```python
from build123d import *

# Parameters (mm, degrees)
CUT_EXTRUDE3_DEPTH           = 60
CUT_EXTRUDE5_DEPTH           = 2
CUT_EXTRUDE5_DEPTH_BACK      = 30
SKETCH9_R                    = 38
SKETCH9_R_2                  = 23
SKETCH19_W                   = 12
SKETCH19_H                   = 36.5
CUT_REVOLVE2_ANGLE           = 65
CUT_REVOLVE2_OTHER_WAY_ANGLE = 65
SKETCH21_W                   = 3.25
SKETCH21_H                   = 4
BOSS_EXTRUDE3_DEPTH          = 1.35
CIRPATTERN1_COUNT            = 5
CUT_EXTRUDE9_START           = -5
CUT_EXTRUDE9_DEPTH           = 5
SKETCH23_R                   = 10.5
CUT_EXTRUDE10_DEPTH          = 10
SKETCH24_W                   = 17
SKETCH24_H                   = 12
BOSS_EXTRUDE4_DEPTH          = 8
SKETCH26_W                   = 12
SKETCH26_H                   = 8
CUT_EXTRUDE11_DEPTH          = 10
SKETCH27_W                   = 4
SKETCH27_H                   = 5
CUT_EXTRUDE12_DEPTH          = 5
CUT_EXTRUDE14_DEPTH          = 2
CUT_EXTRUDE14_DEPTH_BACK     = 30
SKETCH29_R                   = 1
CUT_EXTRUDE15_DEPTH          = 15
FILLET1_R                    = 6
FILLET2_R                    = 8


# Read off the part's stored shape, not the designer's step: Cut-Extrude9
with BuildPart() as part:
    # Sketch1 → Revolve1 (revolve)
    with BuildSketch(Plane.XY, mode=Mode.PRIVATE) as revolve1_sk:
        with BuildLine():
            Line((0, 63.427876097), (32, 63.427876097))
            ThreePointArc((32, 63.427876097), (37.656854249, 61.084730346), (40, 55.427876097))
            Line((40, 55.427876097), (40, 28.846818009))
            ThreePointArc((40, 28.846818009), (38.792081772, 24.082439968), (35.460140376, 20.469057744))
            Line((35.460140376, 20.469057744), (28.539859624, 15.958818353))
            ThreePointArc((28.539859624, 15.958818353), (25.207918228, 12.345436129), (24, 7.581058088))
            Line((24, 7.581058088), (24, 3.25))
            Line((24, 3.25), (24.35, 3))
            Line((24.35, 3), (24.35, 0))
            Line((24.35, 0), (22.5, 0))
            Line((22.5, 0), (22.5, 12.5))
            ThreePointArc((22.5, 12.5), (22.353553391, 12.853553391), (22, 13))
            Line((22, 13), (0, 13))
            Line((0, 13), (0, 63.427876097))
        make_face()
    revolve(revolve1_sk.sketch.rotate(Axis((0, 0, 0), (0, 1, 0)), 90), axis=Axis((0, 0, 0), (0, 1, 0)))

    # Sketch11 → Cut-Extrude3 (cut)
    with BuildSketch(Plane(origin=(0, 13, 0), x_dir=(-1, 0, 0), z_dir=(0, -1, 0))):
        with BuildLine():
            Line((-21, 0), (21, 0))
            ThreePointArc((21, 0), (0, 21), (-21, 0))
        make_face()
    extrude(amount=-CUT_EXTRUDE3_DEPTH, mode=Mode.SUBTRACT)

    # Sketch9 → Cut-Extrude5 (cut, two sides: drawn at the far end of the back side and taken through both)
    with BuildSketch(Plane(origin=(0, 55.427876097, 0), x_dir=(1, 0, 0), z_dir=(0, 1, 0)).offset(-CUT_EXTRUDE5_DEPTH_BACK)):
        with Locations(Location((0, 0, 0), (0, 0, 270))):
            Circle(SKETCH9_R)
        with Locations(Location((0, 0, 0), (0, 0, 270))):
            Circle(SKETCH9_R_2, mode=Mode.SUBTRACT)
    extrude(amount=CUT_EXTRUDE5_DEPTH + CUT_EXTRUDE5_DEPTH_BACK, mode=Mode.SUBTRACT)

    # Sketch19 → Cut-Revolve2 (revolve, cut)
    with BuildSketch(Plane(origin=(0, 0, 0), x_dir=(0, 0, -1), z_dir=(1, 0, 0))):
        with Locations((-41.064715832, 37.177876097)):
            Rectangle(SKETCH19_W, SKETCH19_H)
    revolve(axis=Axis((0, 0, 0), (0, 1, 0)), revolution_arc=CUT_REVOLVE2_ANGLE, mode=Mode.SUBTRACT)

    # Sketch19 → Cut-Revolve2 other way (revolve, cut)
    with BuildSketch(Plane(origin=(0, 0, 0), x_dir=(0, 0, -1), z_dir=(1, 0, 0))):
        with Locations((-41.064715832, 37.177876097)):
            Rectangle(SKETCH19_W, SKETCH19_H)
    revolve(axis=Axis((0, 0, 0), (0, -1, 0)), revolution_arc=CUT_REVOLVE2_OTHER_WAY_ANGLE, mode=Mode.SUBTRACT)

    # Sketch21 → Boss-Extrude3 (add)
    with BuildSketch(Plane(origin=(0, 0, 22.5), x_dir=(-1, 0, 0), z_dir=(0, 0, -1))):
        with Locations((0, 2)):
            Rectangle(SKETCH21_W, SKETCH21_H)
    boss_extrude3 = extrude(amount=BOSS_EXTRUDE3_DEPTH)

    # CirPattern1: Boss-Extrude3 ×5 about axis
    cirpattern1_axis = Axis((0, 0, 0), (0, 1, 0))
    for i in range(1, CIRPATTERN1_COUNT):
        add(boss_extrude3.rotate(cirpattern1_axis, i * 360 / CIRPATTERN1_COUNT))

    # Cut-Extrude9 outline → Cut-Extrude9 (cut)
    with BuildSketch(Plane(origin=(0, 63.427876097, 0), x_dir=(1, 0, 0), z_dir=(0, 1, 0)).offset(CUT_EXTRUDE9_START)):
        with BuildLine():
            ThreePointArc((40, 0), (0, 40), (-40, 0))
            Line((-40, 0), (-21, 0))
            ThreePointArc((-21, 0), (0, 21), (21, 0))
            Line((21, 0), (40, 0))
        make_face()
    extrude(amount=CUT_EXTRUDE9_DEPTH, mode=Mode.SUBTRACT)

    # Sketch23 → Cut-Extrude10 (cut)
    with BuildSketch(Plane(origin=(0, 0, -40), x_dir=(-1, 0, 0), z_dir=(0, 0, -1))):
        with Locations((0, 42.137876097)):
            Circle(SKETCH23_R)
    extrude(amount=-CUT_EXTRUDE10_DEPTH, mode=Mode.SUBTRACT)

    # Sketch24 → Boss-Extrude4 (add)
    with BuildSketch(Plane(origin=(0, 58.427876097, 0), x_dir=(1, 0, 0), z_dir=(0, 1, 0))):
        with Locations((0, 30)):
            Rectangle(SKETCH24_W, SKETCH24_H)
    extrude(amount=-BOSS_EXTRUDE4_DEPTH)

    # Sketch26 → Cut-Extrude11 (cut)
    with BuildSketch(Plane(origin=(0, 58.427876097, 0), x_dir=(1, 0, 0), z_dir=(0, 1, 0))):
        with Locations((0, 30)):
            Rectangle(SKETCH26_W, SKETCH26_H)
    extrude(amount=-CUT_EXTRUDE11_DEPTH, mode=Mode.SUBTRACT)

    # Sketch27 → Cut-Extrude12 (cut)
    with BuildSketch(Plane(origin=(8.5, 0, 0), x_dir=(0, 0, -1), z_dir=(1, 0, 0))):
        with Locations((31, 53.927876097)):
            Rectangle(SKETCH27_W, SKETCH27_H)
    extrude(amount=-CUT_EXTRUDE12_DEPTH, mode=Mode.SUBTRACT)

    # Sketch28 → Cut-Extrude14 (cut, two sides: drawn at the far end of the back side and taken through both)
    with BuildSketch(Plane(origin=(0, 55.427876097, 0), x_dir=(1, 0, 0), z_dir=(0, 1, 0)).offset(-CUT_EXTRUDE14_DEPTH_BACK)):
        with BuildLine():
            Line((-22.912878475, -2), (22.912878475, -2))
            ThreePointArc((22.912878475, -2), (0, -23), (-22.912878475, -2))
        make_face()
    extrude(amount=CUT_EXTRUDE14_DEPTH + CUT_EXTRUDE14_DEPTH_BACK, mode=Mode.SUBTRACT)

    # Sketch29 → Cut-Extrude15 (cut)
    with BuildSketch(Plane(origin=(0, 0, 0), x_dir=(-1, 0, 0), z_dir=(0, 0, -1))):
        with Locations((-30.416198487, 60.927876097)):
            Circle(SKETCH29_R)
        with Locations((30.416198487, 60.927876097)):
            Circle(SKETCH29_R)
        with Locations((0, 60.927876097)):
            Circle(SKETCH29_R)
    extrude(amount=-CUT_EXTRUDE15_DEPTH, mode=Mode.SUBTRACT)

    # Fillet1
    fillet1_edges = [part.edges().sort_by_distance(p)[0] for p in [
        (21, 35.713938048, 0),
        (-21, 35.713938048, 0),
    ]]
    fillet(fillet1_edges, radius=FILLET1_R)

    # Fillet2
    fillet2_edges = [part.edges().sort_by_distance(p)[0] for p in [
        (-22.912878475, 41.427876097, 2),
        (22.912878475, 41.427876097, 2),
    ]]
    fillet(fillet2_edges, radius=FILLET2_R)


solid = part.part
```
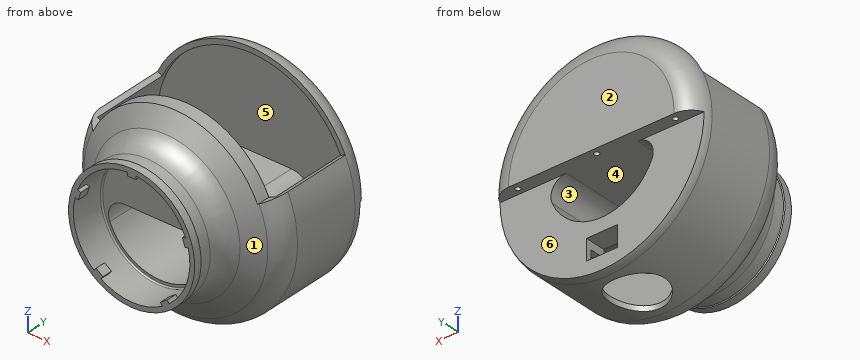
The listing builds one solid part. Answer for the finished solid, in the listing's coordinates (mm). Face numbers are marked on the shaded views. A direction names the side the tool comes from. Coordinates: 2 decimals unless noted, no trailing zeros. Write each loop counter-clockwise with the first axis right and the second up, starting at its lowest first coordinate (ties: lowest second). Pieces come first, ordered by that corner, then holes. Notation, with made-up numbers: (57, -34) - (101, -34) arc R30 ccw to (101, -9) - close; hole circle Ø6 at (57.5, 69). An arc over 180 degrees is marked (long way). Return JSON: item names as keys, results as strings. Group by question number.
Q1. The part is cut by section A-A on y = 22.5. Write down the section's boundary in (x, z), and give its area (3 significant figures).
Q2. The part is cut by section B-B on z = -1.5. State how many separate pieces and enclosed holes the cut face has, and give its area (3 significant figures).
Q3. Find the intervals of material crossed by line 1 along Y through (x, z) = (0, 8); line 2 along Y through (x, z) = (-9.5, 16); line 3 along X through (y, z) = (50, -9), in increasing order. Write a range as [from, to].
Q4. Flat-ended cylindrical pins translate along their axes: pin 1 Ø2 at (x, y) = (0, 61) entering from -Z; pin 2 Ø12 at (x, y) = (-19.5, 28) entering from -Z; pin 3 Ø10 at (x, z) = (2, 2.5) entering from -Y; pin 4 Ø13 at (x, z) = (-2, -27.5) entering from -Y. Find the tip coordinate at first contact, or state that the pin passes through.
Q5. Which of the six approach directions +Z, -Z, +X, -X, +Y, -Y give full straight-line access (tool end or side, diameter ignored) to the marked faces 4, 5 and 6?
Q6. For a pull along Z with two mould halves and no side action, classify the marked faces 1, 2 and 3 as +Z half, -Z half, draft (parallel to the pull), parting line (faces both ways), or undercut.
Evaluation:
{
 "1": {"outline": "(-34.19, 15.94) arc R37.73 ccw (long way) to (34.19, 15.94) - (31.78, 14.82) arc R35.06 ccw to (-31.78, 14.82) - close; hole (-19.25, -8.4) arc R21 ccw to (19.25, -8.4) arc R6 ccw to (13.75, 0) - (-13.75, 0) arc R6 ccw to start", "area": "3,590 mm2"},
 "2": {"separate pieces": "2", "enclosed holes": "2", "area": "768 mm2"},
 "3": {"line 1": "y = [13, 25.43], [57.43, 59.93], [61.93, 63.43]", "line 2": "y = [13, 25.43], [57.43, 63.43]", "line 3": "x = [-38.97, -36.92], [-21.16, -18.97], [18.97, 21.16], [36.92, 38.97]"},
 "4": {"pin 1": "stops at z = 0", "pin 2": "stops at z = -37.64", "pin 3": "stops at y = 13", "pin 4": "stops at y = 0"},
 "5": {"face 4": "+Y", "face 5": "none", "face 6": "-Z, +X, -X, +Y"},
 "6": {"face 1": "parting line", "face 2": "draft", "face 3": "undercut"}
}
